For this review, use the dimensioned drawing (mm, ordinates from the lowest corner) and the shaded views. Give positions to 0.01 mm unless a question says otherwise; leave off trailing zeros. Write each loop counter-clockwise with the first axis right and the second up, starting at its lowest first coordinate (ties: lowest second). Pieces come first, ordered by that corner, then holes. Notation, with made-up numbers: M -20.5,2.25 L 30.5,2.25 A19 ccw 30.5,8.25 Z; hole C 48,4.5 d3. An arc over 180 degrees is marked long. Write each question's results on one line, items separated by ' | '. Start each with the question number.
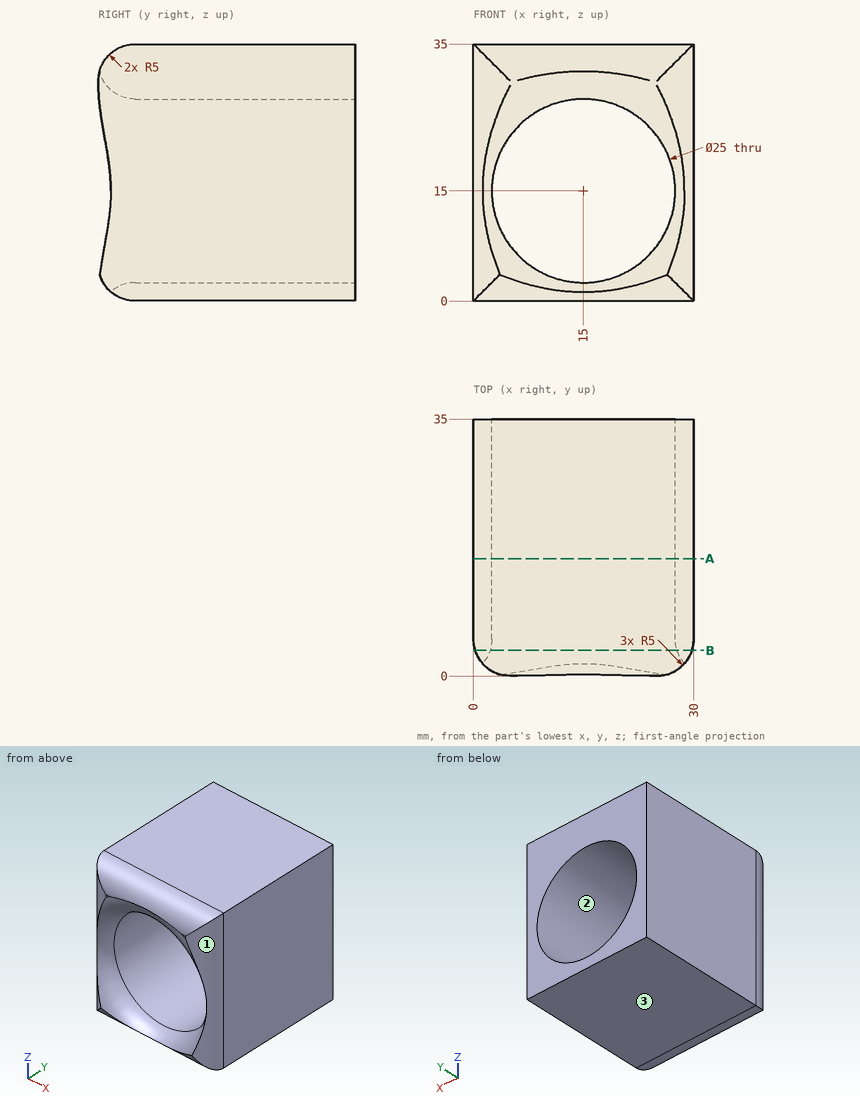
(1) Draft analysis for pull direction X (two halves, no side actions). For the marked faces 1, 2 and 3, state which applies: pulls with the +X half, pulls with the -X half, needs draft (parallel to the pull), parting line crosses it, or undercut.
(2) Add section B-B (y = 3.5). State the section outline as (x, z) points, then the cut area to 3 significant figures.
(3) Add section A-A (y = 16). State the section outline as (x, z) points.
(4) Wall thickness on L1, parallel to Z at x = 15, y = 21; L2, parallel to X at y = 29.5, z = 18; L3, parallel to Z at x = 17, y = 17: over which ranges is each line inside the solid? List them lowest first.
Calculated:
1) face 1: pulls with the +X half | face 2: undercut | face 3: needs draft
2) outline: M 0.23,0.23 L 29.77,0.23 L 29.77,34.77 L 0.23,34.77 Z; hole C 15,15 d25.46 | area: 511 mm²
3) outline: M 0,0 L 30,0 L 30,35 L 0,35 Z; hole C 15,15 d25
4) L1: z = 0 to 2.5, 27.5 to 35 | L2: x = 0 to 2.87, 27.13 to 30 | L3: z = 0 to 2.66, 27.34 to 35
